Geometry check sheet. Reference: the model listing, model coordinates, mm. Coordinates: 2 decimals unless noted, no trailing zeros. Loops run counter-clockwise (first coordinate to the right, second up) from the corner with the lowest first, then second, coordinate; pieces in that order, holes last.
from build123d import *

# Parameters (mm, degrees)
F0_R           = 6.35
F1_DEPTH       = 93.5482
F2_R           = 7.62
F2_R_2         = 3.175
F3_DEPTH       = 12.7
F5_D           = 5.5118
F5_DEPTH       = 50.8
F5_CBORE_D     = 12.7
F5_CBORE_DEPTH = 12.7
F5_TIP         = 1.65591178


with BuildPart() as f1:
    # F0 (on Front) → F1 (new body)
    with BuildSketch(Plane.XZ):
        Circle(F0_R)
    extrude(amount=F1_DEPTH)

    # F2 (on face) → F3 (cut)
    with BuildSketch(Plane.XZ.offset(93.5482)):
        Circle(F2_R)
        Circle(F2_R_2, mode=Mode.SUBTRACT)
    extrude(amount=-F3_DEPTH, mode=Mode.SUBTRACT)

    # F5
    with Locations(Plane(origin=(0, 0, 0), x_dir=(-1, 0, 0), z_dir=(0, 1, 0))):
        with Locations((0, 0)):
            CounterBoreHole(F5_D / 2, F5_CBORE_D / 2, F5_CBORE_DEPTH, depth=F5_DEPTH)
            with Locations((0, 0, -(F5_DEPTH + F5_TIP / 2))):  # 118° drill point
                Cone(0, F5_D / 2, F5_TIP, mode=Mode.SUBTRACT)


solid = f1.part
1) Section check A-A on y = -21. Record the cut outline in (x, z).
Data:
outline: circle Ø12.7 at (0, 0); hole circle Ø5.51 at (0, 0)
2) Depth check by flat-ended pin: pin 1 (1.5 mm diameter, centred on y = -48.5, z = -4, fed in from +X); pin 2 (3 mm diameter, centred on x = 2.5, y = -41, fed in from +Z); pin 3 (1.5 mm diameter, centred on y = -66.5, z = -3.5, fed in from +X). Enter the tip coordinate at first touch or a pass-through.
Data:
pin 1: stops at x = 5.46
pin 2: stops at z = 6.27
pin 3: stops at x = 5.72
3) Section check D-D on z = -5. Record the cut outline in (x, y).
Data:
outline: (-3.91, -80.85) - (3.91, -80.85) - (3.91, -12.7) - (-3.91, -12.7) - close
4) Section check B-B on y = -83.5. Record the cut outline in (x, z) (3 decimals).
Data:
outline: circle Ø6.35 at (0, 0)
5) Section check C-C on x = 4.75. Record the cut outline in (y, z).
Data:
outline: (-80.85, -4.21) - (-12.7, -4.21) - (-12.7, 4.21) - (-80.85, 4.21) - close
6) Mould release check, pull along Z, two halves, no side actions. Record for faces 1 (the cylindrical face through (-0.6, -32.02, -2.69)), 2 (the cylindrical face through (-0.69, -87.29, -3.1)), 3 (the flat face through (-2, -80.848, 3)): +Z half, -Z half, draft (parallel to the pull), parting line (faces both ways), or undercut.
Data:
face 1: undercut
face 2: parting line
face 3: draft
7) Material ranges on probe 1 along Z at (x, y) = (0, -29.5); probe 2 along Y at (x, z) = (2, 2.75), recorded low to high.
Data:
probe 1: z = -6.35 to -2.76, 2.76 to 6.35
probe 2: y = -80.85 to -12.7
